Work out the finished part from the listing and answer in its coordinate system (mm). Face numbers are marked on the shaded views. Coordinates: 2 decimals unless noted, no trailing zeros. Order: outer loops, then holes, each group sorted by start corner. A loop starts at its lowest first (then second) coordinate and runs counter-clockwise, first axis right, second up. Notation, with made-up numbers: (89.5, -30.5) -> (123.5, -30.5) arc R30 ccw to (123.5, 5.5) -> close; hole circle Ø5 at (28.5, 64). An arc over 180 degrees is marked (long way). Use one line per item in the form item = value.
from build123d import *

# Parameters (mm, degrees)
F0_W = 2.032
F0_H = 1.44033
F2_R = 1.27
F3_R = 5.08


with BuildPart() as f1:
    # F0 (on Front) → F1 (revolve)
    with BuildSketch(Plane.XZ):
        Polygon((-49.180098, 5.557153), (-49.180098, 6.35), (-50.292, 6.35), (-50.419, 6.35), (-55.88, 6.35), (-55.88, -6.64733), (-53.34, -6.64733), (-54.102, -4.86933), (-54.102, -1.44033), (-54.102, 0), (-52.07, 0), (-50.546, 0), (-48.416793, 5.557153), align=None)
        Polygon((-54.102, -4.86933), (-53.34, -6.64733), (-52.07, -6.64733), (-52.07, -4.86933), align=None)
        with Locations((-53.086, -0.720165)):
            Rectangle(F0_W, F0_H)
    revolve(axis=Axis((0, 0, 3.175), (0, 0, 1)))

    # F2
    f2_edges = [f1.edges().sort_by_distance(p)[0] for p in [
        (54.102, 0, -1.44033),
        (54.102, 0, -4.86933),
    ]]
    fillet(f2_edges, radius=F2_R)

    # F3
    f3_edges = [f1.edges().sort_by_distance(p)[0] for p in [
        (55.88, 0, 6.35),
    ]]
    fillet(f3_edges, radius=F3_R)


solid = f1.part
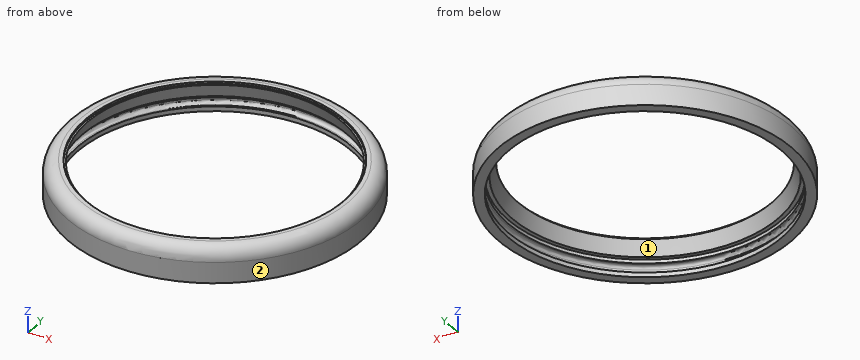
(1) Section C-C on z = 3 is taken. Write down the section's boundary in (x, y).
Data:
outline = circle Ø111.15 at (0, 0); hole circle Ø98.79 at (0, 0)
(2) Each of these flat-tipped pins is pushed along its axis until it touches: P1, Ø4, axis at y = -8, z = -1, coming from the +X side; P2, Ø1.5, axis at y = 42, z = 0.5, coming from the +X side; P3, Ø2, axis at y = -44, z = 0.5, coming from the +X side. Where does it stop, or does it pass through?
Data:
P1 = 55.56
P2 = 37.7
P3 = 35.69
(3) Straight lines are drawn through the part: line 1 along Y through (x, z) = (0, -0.4); line 2 along Y through (x, z) = (0, -3.2). For each, find the intervals that lie inside material, in ascending order.
Data:
line_1 = -55.88 to -52.07, 52.07 to 55.88
line_2 = -55.88 to -54.1, 54.1 to 55.88
(4) The mould has two halves that part along Y. Classify the marked faces 1 and 2: released by +Y, released by -Y, zero draft, split by the parting line, or undercut.
Data:
face_1 = undercut
face_2 = split by the parting line
